The drawing under review shows one solid part. Ordinate dimensions are in mm from its lowest x, y, z. Give positions to 0.01 mm unless a question says otherwise; leave off trailing zeros. Loops run counter-clockwise (first coordinate to the right, second up) from the corner with the lowest first, then second, coordinate; pieces in that order, holes last. Notation, with made-up numbers: M -9,21.5 L -5,21.5 A37 cw -5,59.5 Z; hole C 47.5,41.25 d3. An arc over 180 degrees is marked long. Answer as CSV lines item,"result".
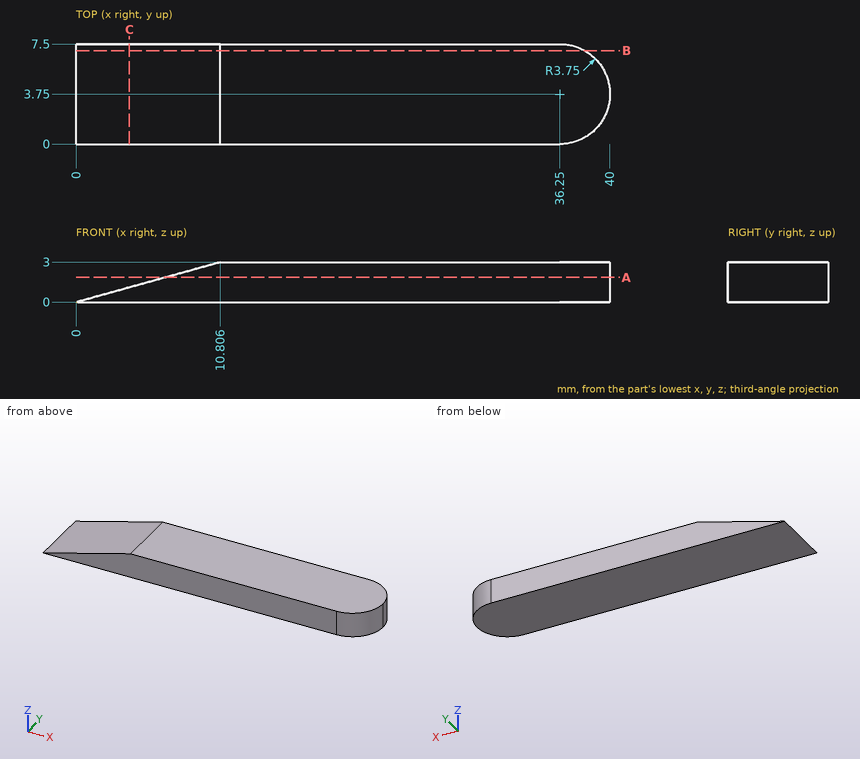
1. For P1, Ø1.5, axis at x = 5.5, z = 0.5, coming from the -Y side, flat-tipped, find the tip position at first contact; note if it passes through.
Answer block:
P1,"y = 0"
2. We need section A-A, the plane z = 1.85. Write out the cut boundary in (x, y).
Answer block:
outline,"M 6.66,0 L 36.25,0 A3.75 ccw 36.25,7.5 L 6.66,7.5 Z"
3. We need section B-B, the plane y = 7. Write out the cut boundary in (x, z).
Answer block:
outline,"M 0,0 L 38.12,0 L 38.12,3 L 10.81,3 Z"
4. We need section C-C, the plane x = 4. Write out the cut boundary in (y, z).
Answer block:
outline,"M 0,0 L 7.5,0 L 7.5,1.11 L 0,1.11 Z"
5. To check wall thickness, follow L1, parallel to Z at x = 10, y = 5; L2, parallel to Z at x = 2, y = 0.5 (1 decimal); L3, parallel to Y at x = 38, z = 0.7. State the ranges of each line that lie inside material, in increasing order. Write a range as [from, to].
Answer block:
L1,"[0, 2.78]"
L2,"[0, 0.6]"
L3,"[0.43, 7.07]"
